```python
from build123d import *

# Parameters (mm, degrees)
F1_DEPTH = 24.13
F2_R     = 7.4295
F3_DEPTH = 54.61
F4_R     = 2.54


with BuildPart() as f1:
    # F0 (on Front) → F1 (new body)
    with BuildSketch(Plane.XZ):
        with BuildLine():
            Line((-7.143751, 47.944095), (-7.143751, 32.704095))
            Line((-7.143751, 32.704095), (12.541249, 32.704095))
            ThreePointArc((12.541249, 32.704095), (27.146249, 47.309095), (41.751249, 32.704095))
            Line((41.751249, 32.704095), (61.436249, 32.704095))
            Line((61.436249, 32.704095), (61.436249, 51.754095))
            Line((61.436249, 51.754095), (-3.333751, 51.754095))
            Line((-3.333751, 51.754095), (-7.143751, 51.754095))
            Line((-7.143751, 51.754095), (-7.143751, 47.944095))
        make_face()
    extrude(amount=F1_DEPTH)

    # F2 (on Top) → F3 (cut)
    with BuildSketch(Plane.XY):
        with Locations((51.49099, -12.054064)):
            Circle(F2_R)
        with Locations((2.793759, -12.054064)):
            Circle(F2_R)
    extrude(amount=F3_DEPTH, mode=Mode.SUBTRACT)

    # F4
    f4_edges = [f1.edges().sort_by_distance(p)[0] for p in [
        (61.436249, 0, 42.229095),
        (-7.143751, 0, 42.229095),
        (-7.143751, -24.13, 42.229095),
        (27.146249, -24.13, 51.754095),
        (27.146249, 0, 51.754095),
        (61.436249, -24.13, 42.229095),
        (-7.143751, -12.065, 51.754095),
        (61.436249, -12.065, 51.754095),
    ]]
    fillet(f4_edges, radius=F4_R)


solid = f1.part
```
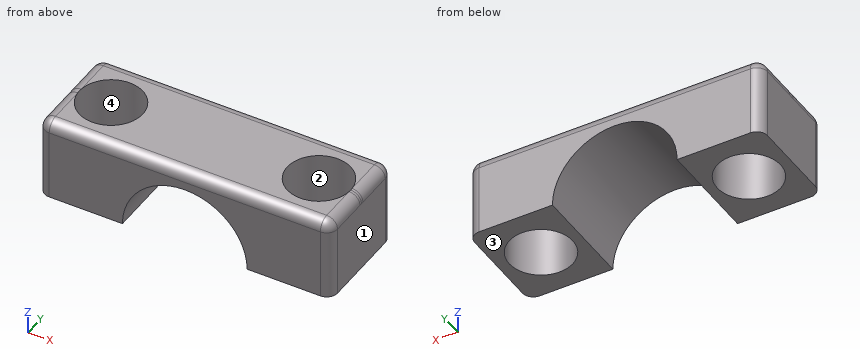
The listing builds one solid part. Answer for the finished solid, in the listing's coordinates (mm). Face numbers are marked on the shaded views. Round coordinates to 2 decimals unless told otherwise and drop trailing zeros. Loops run counter-clockwise (first coordinate to the right, second up) from the corner with the lowest first, then second, coordinate; pieces in that order, holes last.
1) A cutting plane is placed at A-A on z = 40.5. Determine the outline of the cut face in (x, y).
Outcome:
outline: (-7.14, -21.59) arc R2.54 ccw to (-4.6, -24.13) - (14.8, -24.13) - (14.8, 0) - (-4.6, 0) arc R2.54 ccw to (-7.14, -2.54) - close; (39.5, -24.13) - (58.9, -24.13) arc R2.54 ccw to (61.44, -21.59) - (61.44, -2.54) arc R2.54 ccw to (58.9, 0) - (39.5, 0) - close; hole circle Ø14.86 at (2.79, -12.05); hole circle Ø14.86 at (51.49, -12.05)
2) A cutting plane is placed at D-D on x = 4. Determine the outline of the cut face in (y, z), plus the area to 3 significant figures.
Outcome:
outline: (-24.13, 32.7) - (-19.38, 32.7) - (-19.38, 51.75) - (-21.59, 51.75) arc R2.54 ccw to (-24.13, 49.21) - close; (-4.72, 32.7) - (0, 32.7) - (0, 49.21) arc R2.54 ccw to (-2.54, 51.75) - (-4.72, 51.75) - close
area: 178 mm2
3) Given P1, Ø12, axis at x = 2.79, y = -12.05, coming from the -Z side, flat-ended and moving along its own axis, determine where the tip first touches the part or whether it passes through.
Outcome:
P1: passes through
4) A cutting plane is placed at C-C on y = -18. Determine the outline of the cut face in (x, z) (3 decimals), plus the area to 3 significant figures.
Outcome:
outline: (-7.144, 32.704) - (-1.661, 32.704) - (-1.661, 51.754) - (-4.604, 51.754) arc R2.54 ccw to (-7.144, 49.214) - close; (7.248, 32.704) - (12.541, 32.704) arc R14.605 cw to (41.751, 32.704) - (47.036, 32.704) - (47.036, 51.754) - (7.248, 51.754) - close; (55.946, 32.704) - (61.436, 32.704) - (61.436, 49.214) arc R2.54 ccw to (58.896, 51.754) - (55.946, 51.754) - close
area: 629 mm2
5) For a pull along X with two mould halves and no side action, classify the marked faces 1, 2, 3 and 4 as released by +X, released by -X, zero draft, split by the parting line, or undercut.
Outcome:
face 1: released by +X
face 2: undercut
face 3: zero draft
face 4: undercut
6) A cutting plane is placed at B-B on x = 56. Determine the outline of the cut face in (y, z), plus the area to 3 significant figures.
Outcome:
outline: (-24.13, 32.7) - (-17.96, 32.7) - (-17.96, 51.75) - (-21.59, 51.75) arc R2.54 ccw to (-24.13, 49.21) - close; (-6.15, 32.7) - (0, 32.7) - (0, 49.21) arc R2.54 ccw to (-2.54, 51.75) - (-6.15, 51.75) - close
area: 232 mm2
7) Consider line 1 (X direction, y = -12.5, z = 45.5); line 2 (X direction, y = -14.5, z = 44.25); line 3 (X direction, y = -6.5, z = 47.5). Determine where each line is inside the solid, lowest interval first.
Outcome:
line 1: x = -7.14 to -4.62, 10.21 to 20.11, 34.19 to 44.07, 58.91 to 61.44
line 2: x = -7.14 to -4.22, 9.81 to 18.2, 36.09 to 44.48, 58.51 to 61.44
line 3: x = -7.14 to -2.14, 7.73 to 46.56, 56.43 to 61.44
